from build123d import *

# Parameters (mm, degrees)
SKETCH_W     = 180
SKETCH_H     = 180
SKETCH_R     = 2
SKETCH_R_2   = 1.75
SKETCH_R_3   = 2.5
SKETCH_W_2   = 40
SKETCH_H_2   = 40
SKETCH_W_3   = 4
SKETCH_H_3   = 38
PAD_DEPTH    = 3
PAD001_DEPTH = 35
SKETCH002_W  = 22
SKETCH002_H  = 20
POCKET_DEPTH = 200


with BuildPart() as part:
    # Sketch → Pad (new body)
    with BuildSketch(Plane.XY):
        with Locations((90, 90)):
            Rectangle(SKETCH_W, SKETCH_H)
        with Locations((40, 10)):
            Circle(SKETCH_R, mode=Mode.SUBTRACT)
        with Locations((140, 10)):
            Circle(SKETCH_R, mode=Mode.SUBTRACT)
        with Locations((90, 170)):
            Circle(SKETCH_R, mode=Mode.SUBTRACT)
        with Locations((20, 160)):
            Circle(SKETCH_R_2, mode=Mode.SUBTRACT)
        with Locations((78, 160)):
            Circle(SKETCH_R_2, mode=Mode.SUBTRACT)
        with Locations((20, 111)):
            Circle(SKETCH_R_2, mode=Mode.SUBTRACT)
        with Locations((78, 111)):
            Circle(SKETCH_R_2, mode=Mode.SUBTRACT)
        with Locations((90, 25)):
            Circle(SKETCH_R_3, mode=Mode.SUBTRACT)
        with Locations((10, 170)):
            Circle(SKETCH_R_3, mode=Mode.SUBTRACT)
        with Locations((170, 170)):
            Circle(SKETCH_R_3, mode=Mode.SUBTRACT)
        with Locations((129.5, 150)):
            Circle(SKETCH_R_2, mode=Mode.SUBTRACT)
        with Locations((150, 150)):
            Circle(SKETCH_R_2, mode=Mode.SUBTRACT)
        with Locations((129.5, 88.5)):
            Circle(SKETCH_R_2, mode=Mode.SUBTRACT)
        with Locations((150, 88.5)):
            Circle(SKETCH_R_2, mode=Mode.SUBTRACT)
        with Locations((90, 80)):
            Rectangle(SKETCH_W_2, SKETCH_H_2, mode=Mode.SUBTRACT)
        with Locations((129.5, 110.5)):
            Rectangle(SKETCH_W_3, SKETCH_H_3, mode=Mode.SUBTRACT)
        with Locations((150, 110.5)):
            Rectangle(SKETCH_W_3, SKETCH_H_3, mode=Mode.SUBTRACT)
    extrude(amount=PAD_DEPTH)

    # Sketch001 → Pad001 (join)
    with BuildSketch(Plane.XY.offset(3)):
        Polygon((0, 0), (69, 0), (69, 1.75), (66, 1.75), (66, 4.25), (69, 4.25), (69, 18), (66, 18), (66, 6), (6, 6), (6, 52), (66, 52), (66, 40), (69, 40), (69, 55), (0, 55), align=None)
        Polygon((180, 0), (111, 0), (111, 1.75), (114, 1.75), (114, 4.25), (111, 4.25), (111, 18), (114, 18), (114, 6), (174, 6), (174, 52), (114, 52), (114, 40), (111, 40), (111, 55), (180, 55), align=None)
    extrude(amount=PAD001_DEPTH)

    # Sketch002 (on Face10 of Pad001) → Pocket (cut)
    with BuildSketch(Plane.YZ.offset(180)):
        with Locations((29, 28)):
            Rectangle(SKETCH002_W, SKETCH002_H)
    extrude(amount=-POCKET_DEPTH, mode=Mode.SUBTRACT)


solid = part.part
Model file for the job. Use its own axes, mm. A direction names the side the tool comes from. Give positions to 0.01 mm unless a question says otherwise; leave off trailing zeros. Order: outer loops, then holes, each group sorted by start corner. A loop starts at its lowest first (then second) coordinate and runs counter-clockwise, first axis right, second up. Notation, with made-up numbers: (-8, -10) - (5, -10) arc R9 ccw to (5, -2) - close; hole circle Ø2 at (14, 84.25). An arc over 180 degrees is marked (long way). Write item = value, one per line. Start each with the question number.
1. Cut at C-C, the plane y = 25. List the corners of the cut face in (x, z).
2. Probe line 1 along Y through (x, z) = (150, 1.55); line 2 along X through (y, z) = (170, 1.6); line 3 along Y through (x, z) = (90, 1). List the from-to ranges inside material, lowest first.
3. Cut at B-B, the plane x = 95. List the corners of the cut face in (y, z), and give its area (3 significant figures).
4. Drop flat-ended pins along their axis: P1, Ø4.5, axis at x = 78, y = 111, coming from the +Z side; P2, Ø6, axis at x = 27, z = 7.5, coming from the +Y side. Give the stop position or say it passes through.
5. Cut at D-D, the plane x = 30.5. List the corners of the cut face in (y, z), and give its area (3 significant figures).
6. Which spindle directions (+Z, -Z, +X, -X, +Y, -Y) get a long thin tool onto all of the face, cutting with end or side? Do faces 1 (the flat face through (111, 47, 20)), 2 (the flat face through (36, 52, 20)), 3 (the flat face through (89, 0, 2)), 4 (the flat face through (177, 18, 28)). Say none if no direction does.
Taken from the geometry:
q1.outline = (0, 0) - (87.5, 0) - (87.5, 3) - (6, 3) - (6, 18) - (0, 18) - close; (92.5, 0) - (180, 0) - (180, 18) - (174, 18) - (174, 3) - (92.5, 3) - close
q2.line_1 = 0 to 86.75, 90.25 to 91.5, 129.5 to 148.25, 151.75 to 180
q2.line_2 = 0 to 7.5, 12.5 to 88, 92 to 167.5, 172.5 to 180
q2.line_3 = 0 to 22.5, 27.5 to 60, 100 to 168, 172 to 180
q3.outline = (0, 0) - (60, 0) - (60, 3) - (0, 3) - close; (100, 0) - (180, 0) - (180, 3) - (100, 3) - close
q3.area = 420 mm²
q4.P1 = 3
q4.P2 = 55
q5.outline = (0, 0) - (180, 0) - (180, 3) - (55, 3) - (55, 38) - (52, 38) - (52, 3) - (6, 3) - (6, 38) - (0, 38) - close
q5.area = 855 mm²
q6.face_1 = +Z, +Y, -Y
q6.face_2 = +Z
q6.face_3 = +Z, -Z, +X, -X, -Y
q6.face_4 = +Z, +X, -X
